Read the model definition and answer for the solid it produces. Units are mm, in the model's axes. A direction names the side the tool comes from. Give positions to 0.01 mm unless a question says otherwise; leave off trailing zeros. Order: outer loops, then holes, each group sorted by start corner. A loop starts at its lowest first (then second) coordinate and runs counter-clockwise, first axis right, second up. Notation, with made-up numbers: (46.25, 13.25) - (83.25, 13.25) arc R30 ccw to (83.25, 50.25) - close; hole circle Ø6 at (11.25, 21.25). An arc over 180 degrees is marked (long way). Use a Markdown table: item, result. Add a question column.
1. A cutting plane is placed at D-D on z = 86. Determine the outline of the cut face in (x, y).
2. Consider L1, parallel to X at y = -121, z = 66; L2, parallel to Z at x = 226, y = 78.5; L3, parallel to X at y = -8, z = 334.5. Determine where each line is inside the solid, lowest interval first.
3. A cutting plane is placed at C-C on y = 4.5. Determine the outline of the cut face in (x, z), and give its area (3 significant figures).
4. Which of the six approach directions +Z, -Z, +X, -X, +Y, -Y give full straight-line access (tool end or side, diameter ignored) to faces 4 (the flat face through (-257, -2, 164)), 5 (the flat face through (275, -2, 222))?
5. For a pull along X with two mould halves and no side action, classify faces 1 (the flat face through (-275, -2, 222)), 2 (the flat face through (-135, 2, 314)), 3 (the flat face through (1, 150, 224)) as released by +X, released by -X, zero draft, split by the parting line, or undercut.
6. A cutting plane is placed at A-A on z = 381. Determine the outline of the cut face in (x, y).
7. A cutting plane is placed at B-B on x = 103. Determine the outline of the cut face in (y, z).
```python
from build123d import *

# Parameters (mm, degrees)
F0_W     = 550
F0_H     = 300
F1_DEPTH = 18
F2_W     = 18
F2_H     = 300
F3_DEPTH = 414
F4_W     = 18
F4_H     = 300
F5_DEPTH = 296
F6_W     = 248
F6_H     = 300
F6_W_2   = 18
F7_DEPTH = 18
F8_W     = 532
F8_H     = 300
F8_W_2   = 18
F9_DEPTH = 18


with BuildPart() as f1:
    # F0 (on Top) → F1 (new body)
    with BuildSketch(Plane.XY):
        Rectangle(F0_W, F0_H)
    extrude(amount=F1_DEPTH)

    # F2 (on face) → F3 (join)
    with BuildSketch(Plane.XY.offset(18)):
        with Locations((-266, 0)):
            Rectangle(F2_W, F2_H)
        with Locations((266, 0)):
            Rectangle(F2_W, F2_H)
    extrude(amount=F3_DEPTH)

    # F4 (on face) → F5 (join)
    with BuildSketch(Plane.XY.offset(18)):
        Rectangle(F4_W, F4_H)
    extrude(amount=F5_DEPTH)

    # F6 (on face) → F7 (join)
    with BuildSketch(Plane.XY.offset(314)):
        with Locations((133, 0)):
            Rectangle(F6_W, F6_H)
        Rectangle(F6_W_2, F6_H)
        with Locations((-133, 0)):
            Rectangle(F6_W, F6_H)
    extrude(amount=F7_DEPTH)

    # F8 (on face) → F9 (join)
    with BuildSketch(Plane.XY.offset(432)):
        with Locations((9, 0)):
            Rectangle(F8_W, F8_H)
        with Locations((-266, 0)):
            Rectangle(F8_W_2, F8_H)
    extrude(amount=F9_DEPTH)


solid = f1.part
```
Output values:
| question | item | result |
|---|---|---|
| 1 | outline | (-275, -150) - (-257, -150) - (-257, 150) - (-275, 150) - close; (-9, -150) - (9, -150) - (9, 150) - (-9, 150) - close; (257, -150) - (275, -150) - (275, 150) - (257, 150) - close |
| 2 | L1 | -275 to -257, -9 to 9, 257 to 275 |
| 2 | L2 | 0 to 18, 314 to 332, 432 to 450 |
| 2 | L3 | -275 to -257, 257 to 275 |
| 3 | outline | (-275, 0) - (275, 0) - (275, 450) - (-275, 450) - close; hole (-257, 18) - (-9, 18) - (-9, 314) - (-257, 314) - close; hole (-257, 332) - (257, 332) - (257, 432) - (-257, 432) - close; hole (9, 18) - (257, 18) - (257, 314) - (9, 314) - close |
| 3 | area | 49,300 mm² |
| 4 | face 4 | +Y, -Y |
| 4 | face 5 | +Z, -Z, +X, +Y, -Y |
| 5 | face 1 | released by -X |
| 5 | face 2 | undercut |
| 5 | face 3 | zero draft |
| 6 | outline | (-275, -150) - (-257, -150) - (-257, 150) - (-275, 150) - close; (257, -150) - (275, -150) - (275, 150) - (257, 150) - close |
| 7 | outline | (-150, 0) - (150, 0) - (150, 18) - (-150, 18) - close; (-150, 314) - (150, 314) - (150, 332) - (-150, 332) - close; (-150, 432) - (150, 432) - (150, 450) - (-150, 450) - close |
